Geometry check sheet. Reference: the model listing, model coordinates, mm. A direction names the side the tool comes from. Give positions to 0.01 mm unless a question says otherwise; leave off trailing zeros. Loops run counter-clockwise (first coordinate to the right, second up) from the corner with the lowest first, then second, coordinate; pieces in that order, holes last. Notation, with made-up numbers: (-35.5, 71.5) -> (-25.5, 71.5) arc R29 cw to (-25.5, 108.5) -> close; hole circle Ø6 at (-12.75, 22.25). An arc over 180 degrees is marked (long way). Write item = value, one per line.
```python
from build123d import *

# Parameters (mm, degrees)
SALIENTE_EXTRUIR1_DEPTH = 196
VACIADO1_T              = -4
CROQUIS2_R              = 8.2
CORTAR_EXTRUIR1_DEPTH   = 4
CROQUIS3_R              = 9.2
CROQUIS3_R_2            = 8.2
SALIENTE_EXTRUIR2_DEPTH = 9
REDONDEO3_R             = 3
REDONDEO4_R             = 3
CORTAR_EXTRUIR2_REACH   = 229.294
CROQUIS4_R              = 8.2
CROQUIS5_R              = 9.2
CROQUIS5_R_2            = 8.2
SALIENTE_EXTRUIR3_DEPTH = 43
CROQUIS6_W              = 82.873764354
CROQUIS6_H              = 43.688886644
CORTAR_EXTRUIR3_DEPTH   = 21.855248
CORTAR_EXTRUIR4_REACH   = 229.294
CROQUIS9_W              = 20
CROQUIS9_H              = 3


with BuildPart() as part:
    # Croquis1 → Saliente-Extruir1 (new body)
    with BuildSketch(Plane(origin=(0, 0, 0), x_dir=(0, 0, -1), z_dir=(1, 0, 0))):
        Polygon((0, 0), (105.85, 0), (105.85, 45.19), (53.855344849, 45.19), align=None)
    extrude(amount=SALIENTE_EXTRUIR1_DEPTH)

    # Vaciado1
    vaciado1_openings = [part.faces().sort_by_distance(p)[0] for p in [
        (98, 0, -52.925),
    ]]
    offset(amount=VACIADO1_T, openings=vaciado1_openings, kind=Kind.INTERSECTION)

    # Croquis2 → Cortar-Extruir1 (cut)
    with BuildSketch(Plane(origin=(196, 0, 0), x_dir=(0, 0, -1), z_dir=(1, 0, 0))):
        with Locations((48.192305519, 14.33)):
            Circle(CROQUIS2_R)
        with Locations((74.192305519, 14.33)):
            Circle(CROQUIS2_R)
    cortar_extruir1 = extrude(amount=-CORTAR_EXTRUIR1_DEPTH, mode=Mode.SUBTRACT)

    # Croquis3 → Saliente-Extruir2 (add)
    # profile 1 of 2: a face of its own
    with BuildSketch(Plane(origin=(196, 0, 0), x_dir=(0, 0, -1), z_dir=(1, 0, 0))):
        with Locations((48.192305519, 14.33)):
            Circle(CROQUIS3_R)
        with Locations((48.192305519, 14.33)):
            Circle(CROQUIS3_R_2, mode=Mode.SUBTRACT)
    # profile 2 of 2: a face of its own
    with BuildSketch(Plane(origin=(196, 0, 0), x_dir=(0, 0, -1), z_dir=(1, 0, 0))):
        with Locations((74.192305519, 14.33)):
            Circle(CROQUIS3_R)
        with Locations((74.192305519, 14.33)):
            Circle(CROQUIS3_R_2, mode=Mode.SUBTRACT)
    saliente_extruir2 = extrude(amount=-SALIENTE_EXTRUIR2_DEPTH)

    # Redondeo3
    redondeo3_edges = [part.edges().sort_by_distance(p)[0] for p in [
        (192, 14.33, -38.992305519),
        (192, 14.33, -64.992305519),
    ]]
    fillet(redondeo3_edges, radius=REDONDEO3_R)

    # Simetría1: Cortar-Extruir1, Saliente-Extruir2 across plane
    add(cortar_extruir1.mirror(Plane(origin=(98, 0, 0), x_dir=(0, 0, 1), z_dir=(1, 0, 0))), mode=Mode.SUBTRACT)
    add(saliente_extruir2.mirror(Plane(origin=(98, 0, 0), x_dir=(0, 0, 1), z_dir=(1, 0, 0))))

    # Redondeo4
    redondeo4_edges = [part.edges().sort_by_distance(p)[0] for p in [
        (4, 14.33, -38.992305519),
        (4, 14.33, -64.992305519),
    ]]
    fillet(redondeo4_edges, radius=REDONDEO4_R)

    # Cortar-Extruir2: up to this plane
    cortar_extruir2_end = Plane(origin=(196, -3.064177772, -2.571150439), z_dir=(0, -0.7660444431189772, -0.6427876096865404))
    # Croquis4 → Cortar-Extruir2 (cut, up to the surface)
    with BuildSketch(Plane.XY, mode=Mode.PRIVATE) as cortar_extruir2_sk1:
        with Locations(Location((85, 19.33, 0), (0, 0, 270))):
            Circle(CROQUIS4_R)
    cortar_extruir2_tool1 = split(extrude(cortar_extruir2_sk1.sketch, amount=-CORTAR_EXTRUIR2_REACH, mode=Mode.PRIVATE), bisect_by=cortar_extruir2_end, keep=Keep.BOTH, mode=Mode.PRIVATE)
    add(cortar_extruir2_tool1.solids().sort_by_distance((85, 19.33, 0))[0], mode=Mode.SUBTRACT)
    # Croquis4 → Cortar-Extruir2 (cut, up to the surface)
    with BuildSketch(Plane.XY, mode=Mode.PRIVATE) as cortar_extruir2_sk2:
        with Locations(Location((111, 19.33, 0), (0, 0, 270))):
            Circle(CROQUIS4_R)
    cortar_extruir2_tool2 = split(extrude(cortar_extruir2_sk2.sketch, amount=-CORTAR_EXTRUIR2_REACH, mode=Mode.PRIVATE), bisect_by=cortar_extruir2_end, keep=Keep.BOTH, mode=Mode.PRIVATE)
    add(cortar_extruir2_tool2.solids().sort_by_distance((111, 19.33, 0))[0], mode=Mode.SUBTRACT)

    # Croquis5 → Saliente-Extruir3 (add)
    # profile 1 of 2: a face of its own
    with BuildSketch(Plane.XY):
        with Locations((111, 19.33)):
            Circle(CROQUIS5_R)
        with Locations((111, 19.33)):
            Circle(CROQUIS5_R_2, mode=Mode.SUBTRACT)
    # profile 2 of 2: a face of its own
    with BuildSketch(Plane.XY):
        with Locations((85, 19.33)):
            Circle(CROQUIS5_R)
        with Locations((85, 19.33)):
            Circle(CROQUIS5_R_2, mode=Mode.SUBTRACT)
    extrude(amount=-SALIENTE_EXTRUIR3_DEPTH)

    # Croquis6 → Cortar-Extruir3 (cut)
    with BuildSketch(Plane(origin=(0, 0, 0), x_dir=(1, 0, 0), z_dir=(0, 0.7660444431189771, 0.6427876096865404))):
        with Locations((99.35120268, 26.550188106)):
            Rectangle(CROQUIS6_W, CROQUIS6_H)
    extrude(amount=CORTAR_EXTRUIR3_DEPTH, mode=Mode.SUBTRACT)

    # Croquis9 → Cortar-Extruir4 (cut, up to next)
    with BuildSketch(Plane(origin=(0, 45.19, 0), x_dir=(1, 0, 0), z_dir=(0, 1, 0)), mode=Mode.PRIVATE) as cortar_extruir4_sk1:
        with Locations((98, 63.355344849)):
            Rectangle(CROQUIS9_W, CROQUIS9_H)
    cortar_extruir4_tool1 = extrude(cortar_extruir4_sk1.sketch, amount=-CORTAR_EXTRUIR4_REACH, mode=Mode.PRIVATE) & part.part
    add(cortar_extruir4_tool1.solids().sort_by_distance((98, 45.19, -63.355345))[0], mode=Mode.SUBTRACT)


solid = part.part
```
Item 1: Draft check along X on faces 1 (the flat face through (196, 23, -64)), 2 (the flat face through (77, 16, -43)), 3 (the flat face through (97, 22, -105.85)). Enter one of: +X half, -X half, draft (parallel to the pull), parting line (faces both ways), or undercut.
Answer:
face_1 = +X half
face_2 = undercut
face_3 = draft
Item 2: Section check B-B, the plane x = 123.5. Record the cut outline in (y, z).
Answer:
outline = (0, -105.85) -> (45.19, -105.85) -> (45.19, -53.86) -> (0, 0) -> (0, -6.22) -> (41.19, -55.31) -> (41.19, -101.85) -> (0, -101.85) -> close
Item 3: Tool access check on faces 4 (the cylindrical face through (4.4, 14.7, -40)), 5 (the cylindrical face through (83.006, 10.349, -33.22)), 6 (the flat face through (98, 43, -64.855)), 7 (the flat face through (103, 16, -43)). Record the directions out of +Z, -Z, +X, -X, +Y, -Y that give a thin tool (end or side, any length) a straight path to the whole face; none if there is none.
Answer:
face_4 = -X
face_5 = none
face_6 = +Y, -Y
face_7 = -Y
Item 4: Section check D-D, the plane y = 17. Give the number of separate pieces and of enclosed holes in the cut face, plus the area to 3 significant figures.
Answer:
separate_pieces = 6
enclosed_holes = 0
area = 2,290 mm^2
Item 5: Thickness scan on L1, parallel to X at y = 19, z = -25; L2, parallel to X at y = 3, z = -28; L3, parallel to X at y = 5.5, z = -75. Record the ranges inside material, lowest first. Write a range as [from, to].
Answer:
L1 = [0, 76.81], [93.19, 102.81], [119.19, 196]
L2 = [0, 4], [192, 196]
L3 = [0, 9], [187, 196]
Item 6: Gauge pin test, flat ends, axial feed: pin 1 (10 mm diameter, centred on x = 82.5, z = -35.5, fed in from -Y); pin 2 (20.5 mm diameter, centred on x = 114.5, y = 26.5, fed in from +Z); pin 3 (8 mm diameter, centred on x = 81, z = -35.5, fed in from +Y); pin 4 (10 mm diameter, centred on y = 14.33, z = -74.19, fed in from +X). Record the tip position at first contact, or that the pin passes through.
Answer:
pin_1 = 10.13
pin_2 = -20.57
pin_3 = 33.14
pin_4 = through
Item 7: Section check A-A, the plane y = 35.5. Record the cut outline in (x, z).
Answer:
outline = (0, -105.85) -> (196, -105.85) -> (196, -42.31) -> (0, -42.31) -> close; hole (4, -101.85) -> (192, -101.85) -> (192, -48.53) -> (4, -48.53) -> close
Item 8: Section check C-C, the plane x = 85. Record the cut outline in (y, z), plus the area to 3 significant figures.
Answer:
outline = (0, -105.85) -> (45.19, -105.85) -> (45.19, -53.86) -> (27.53, -32.81) -> (27.53, -43) -> (28.53, -43) -> (28.53, -40.22) -> (41.19, -55.31) -> (41.19, -101.85) -> (0, -101.85) -> close; (0, -6.22) -> (10.13, -18.3) -> (10.13, -43) -> (11.13, -43) -> (11.13, -13.26) -> (0, 0) -> close
area = 564 mm^2
